Job drawing, mm, ordinate dimensions from the low corner. One solid piece. A direction names the side the tool comes from. Round coordinates to 2 decimals unless told otherwise and drop trailing zeros. Loops run counter-clockwise (first coordinate to the right, second up) from the corner with the lowest first, then second, coordinate; pieces in that order, holes last. Notation, with made-up numbers: M -22.75,73.5 L -7.75,73.5 A7 cw -7.75,83.5 Z; hole C 18,53 d8. An arc over 180 degrees is marked long. Use one line per item in the form item = value.
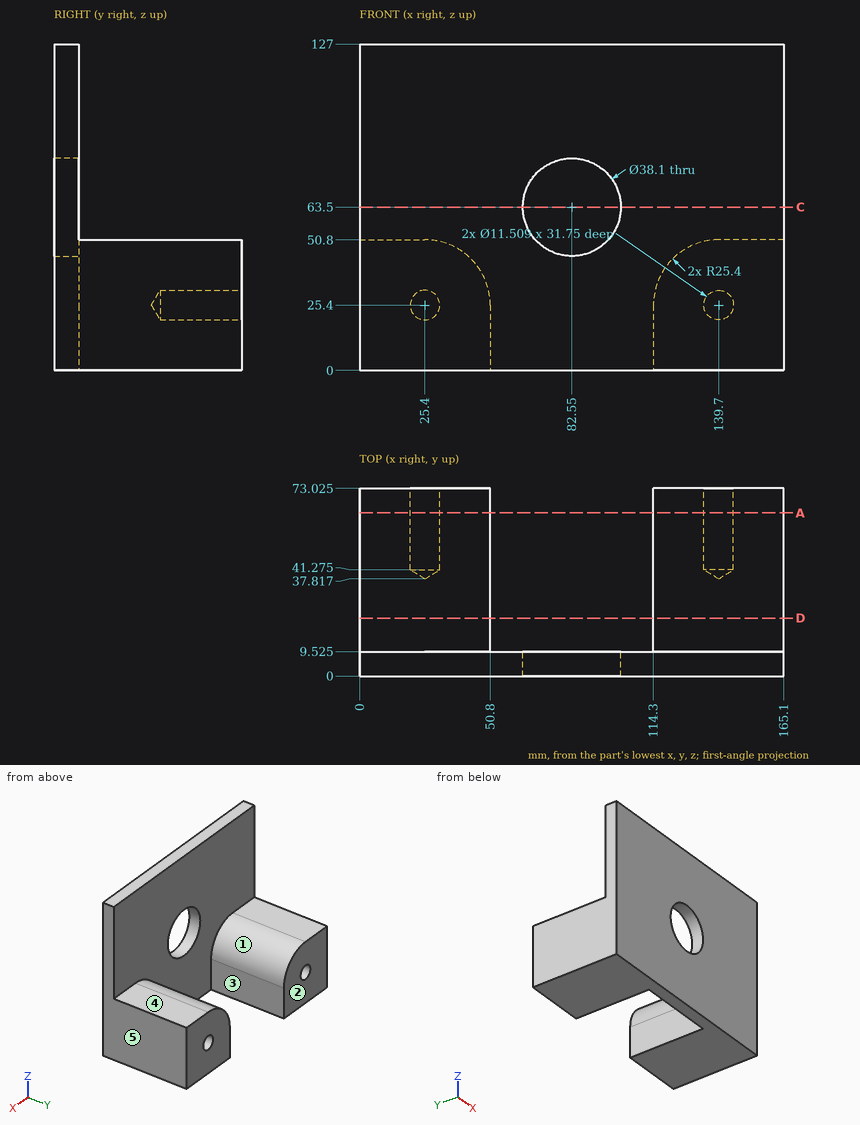
1. Cut at C-C on z = 63.5. Write the cut outline in (x, y) (1 decimal).
Completed:
outline = M 0,0 L 63.5,0 L 63.5,9.5 L 0,9.5 Z; M 101.6,0 L 165.1,0 L 165.1,9.5 L 101.6,9.5 Z
2. Cut at D-D on y = 22.5. Write the cut outline in (x, z), and give its area (3 significant figures).
Completed:
outline = M 0,0 L 50.8,0 L 50.8,25.4 A25.4 ccw 25.4,50.8 L 0,50.8 Z; M 114.3,0 L 165.1,0 L 165.1,50.8 L 139.7,50.8 A25.4 ccw 114.3,25.4 Z
area = 4,880 mm2
3. Cut at A-A on y = 63.5. Write the cut outline in (x, z) (1 decimal).
Completed:
outline = M 0,0 L 50.8,0 L 50.8,25.4 A25.4 ccw 25.4,50.8 L 0,50.8 Z; M 114.3,0 L 165.1,0 L 165.1,50.8 L 139.7,50.8 A25.4 ccw 114.3,25.4 Z; hole C 25.4,25.4 d11.5; hole C 139.7,25.4 d11.5
4. Tool access for the marked faces 1, 2, 3, 4 and 5: list every direction of +Z, -Z, +X, -X, +Y, -Y with a clear straight run to the whole face (end or side of a thin tool).
Completed:
face_1 = +Z, +Y
face_2 = +Z, -Z, +X, -X, +Y
face_3 = +Z, -Z, +Y
face_4 = +Z, +X, -X, +Y
face_5 = +Z, -Z, +X, +Y, -Y
5. Drop flat-ended pins along their axis: P1, Ø6, axis at x = 20, z = 114.5, coming from the +Y side (3 decimals); P2, Ø7, axis at x = 25.4, z = 25.4, coming from the +Y side; P3, Ø8, axis at x = 116.5, y = 38.5, coming from the +Z side. Give the stop position or say it passes through.
Completed:
P1 = 9.525
P2 = 39.92
P3 = 42.03
6. Probe line 1 along X through (y, z) = (66, 25); line 2 along X through (y, z) = (3, 63.5); line 3 along Z through (x, y) = (82, 2). List the from-to ranges inside material, lowest first. Write a range as from..to.
Completed:
line_1 = 0..19.66, 31.14..50.8, 114.3..133.96, 145.44..165.1
line_2 = 0..63.5, 101.6..165.1
line_3 = 0..44.46, 82.54..127
